Answer from the drawing. Dimensions are ordinates in mm from the lowest x, y and z of the part. Give positions to 0.01 mm unless a question says otherwise; leave off trailing zeros. Order: outer loops, then holes, each group sorted by start corner. A loop starts at its lowest first (then second) coordinate and runs counter-clockwise, first axis right, second up.
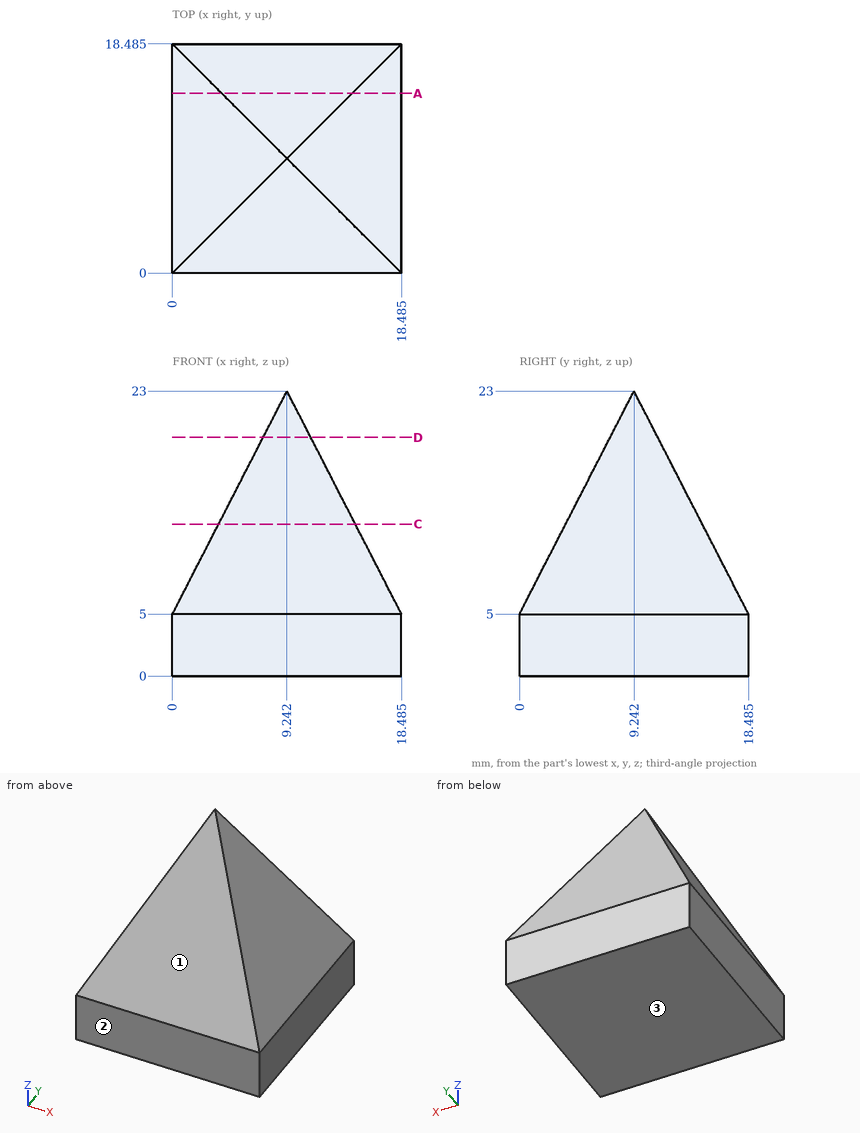
1. The part is cut by section A-A (y = 14.5). Write down the section's boundary in (x, z) (1 decimal), then the cut area to 3 significant figures.
Findings below:
outline: (0, 0) - (18.5, 0) - (18.5, 5) - (14.5, 12.8) - (4, 12.8) - (0, 5) - close
area: 205 mm2
2. The part is cut by section C-C (z = 12.25). Write down the section's boundary in (x, y).
Findings below:
outline: (3.72, 3.72) - (14.76, 3.72) - (14.76, 14.76) - (3.72, 14.76) - close
3. Given P1, Ø8, axis at y = 7.5, z = 8.5, coming from the +X side (1 decimal); P2, Ø2, axis at x = 16, z = 8, coming from the -Y side; P3, Ø4, axis at x = 12.5, y = 8.5, coming from the +Z side; P4, Ø6, axis at x = 15, y = 2.5, coming from the +Z side (1 decimal), each flat-ended and moving along its own axis, determine where each tip first touches the part or whether it passes through.
Findings below:
P1: stops at x = 18.5
P2: stops at y = 1.03
P3: stops at z = 20.55
P4: stops at z = 14.8
4. The mould has two halves that part along Z. Classify the marked faces 1, 2 and 3: pulls with the +Z half, pulls with the -Z half, needs draft (parallel to the pull), parting line crosses it, or undercut.
Findings below:
face 1: pulls with the +Z half
face 2: needs draft
face 3: pulls with the -Z half
5. The part is cut by section D-D (z = 19.25). Write down the section's boundary in (x, y), then the cut area to 3 significant figures.
Findings below:
outline: (7.32, 7.32) - (11.17, 7.32) - (11.17, 11.17) - (7.32, 11.17) - close
area: 14.8 mm2
6. Straight lines are drawn through the part: probe 1 along Z at (x, y) = (13, 15.5) (1 decimal); probe 2 along Y at (x, z) = (12.25, 6.5) (1 decimal); probe 3 along Z at (x, y) = (14.25, 4). For each, find the intervals that lie inside material, in ascending order.
Findings below:
probe 1: z = 0 to 10.8
probe 2: y = 0.8 to 17.7
probe 3: z = 0 to 12.79
